Autodesk Inventor part; units mm, degrees
ref_plane "YZ Plane" through (0, 0, 0) normal (1, 0, 0) x (0, 1, 0)
ref_plane "XZ Plane" through (0, 0, 0) normal (0, 1, 0) x (-1, 0, 0)
ref_plane "XY Plane" through (0, 0, 0) normal (0, 0, 1) x (1, 0, 0)
sketch "Boceto1" plane through (0, 0, 0) normal (0, 0, 1) x (1, 0, 0)
  line L0 (0, 26.9924) -> (5, 26.9924)
  arc A0 (5, 26.9924) -> (5.5, 27.4924) centre (5, 27.4924) ccw
  line L1 (5.5, 27.4924) -> (5.5, 36.4924)
  arc A1 (6, 36.9924) -> (5.5, 36.4924) centre (6, 36.4924) ccw
  line L2 (6, 36.9924) -> (9.9731, 36.9924)
  arc A2 (10.4724, 36.4662) -> (9.9731, 36.9924) centre (9.9731, 36.4924) ccw
  line L3 (10.4724, 36.4662) -> (10.0035, 27.5185)
  arc A3 (10.0035, 27.5185) -> (10.5028, 26.9924) centre (10.5028, 27.4924) ccw
  arc A4 (23, -23.0504) -> (54.0922, -16.3077) centre (23, 52.0085) ccw
  arc A5 (106.311, -20.6517) -> (54.0922, -16.3077) centre (76.3195, -65.146) ccw
  arc A6 (106.311, -20.6517) -> (116.3303, -5.6981) centre (111.3414, -13.1888) ccw
  arc A7 (106.3579, 7.7696) -> (116.3303, -5.6981) centre (130.0298, 14.8719) ccw
  arc A8 (106.3579, 7.7696) -> (102.827, 7.7277) centre (104.6036, 6.8117) ccw
  line L4 (102.827, 7.7277) -> (98.8026, -0.0781)
  arc A9 (96.3676, -1.0494) -> (98.8026, -0.0781) centre (97.026, 0.8379) ccw
  arc A10 (96.3676, -1.0494) -> (30.1711, -1.1614) centre (63.429, -95.4689) ccw
  line L5 (13.5421, 45.9924) -> (0, 45.9924)
  arc A11 (0, 45.9924) -> (-1.9988, 43.9936) centre (0, 43.9936) ccw
  line L6 (-1.9988, 43.9936) -> (-1.9988, 28.9912)
  arc A12 (-1.9988, 28.9912) -> (0, 26.9924) centre (0, 28.9912) ccw
  circle A13 centre (111.3414, -13.1888) radius 1.9988
  circle A14 centre (31.3414, -9.1385) radius 1.9988
  line L7 (10.5028, 26.9924) -> (10.5028, -23.0504)
  line L8 (23, -23.0504) -> (13.5421, -23.0504)
  line L9 (13.5421, 45.9924) -> (27.5683, 45.9924)
  line L10 (27.5683, 45.9924) -> (27.5683, -2)
  arc A15 (27.5683, -2) -> (30.1711, -1.1614) centre (13.5421, 45.9924) ccw
  line L11 (13.5421, -23.0504) -> (10.5028, -23.0504)
  point P0 (0, 0)
extrude "Extrusión2" add sketch "Boceto1" along normal blind 5
fillet "Empalme1" radius 2 3 edges at (10.5028, -23.0504, 2.5) (27.5683, 45.9924, 2.5) (27.5683, -2, 2.5)
properties part number "soporte bobina nuevo"
Geometry check sheet. Reference: the model listing, model coordinates, mm. A direction names the side the tool comes from. Coordinates: 2 decimals unless noted, no trailing zeros. Order: outer loops, then holes, each group sorted by start corner. A loop starts at its lowest first (then second) coordinate and runs counter-clockwise, first axis right, second up. Notation, with made-up numbers: (58, 37.5) - (62, 37.5) arc R25 ccw to (62, 65.5) - close; hole circle Ø4 at (72, -37). An arc over 180 degrees is marked (long way). Answer as a JSON object with one key per item and string values. Group by question number.
Item 1: Sectioned sample at A-A, the plane y = 6.5. Record the cut outline in (x, z).
Item 2: Tool access check on faces 4 (the face through (27.568, 23, 2)), 5 (the face through (5.5, 32, 2)), 6 (the face through (10.24, 32.05, 2.46)), 7 (the face through (2, 26.992, 2)). Record the directions out of +Z, -Z, +X, -X, +Y, -Y that give a thin tool (end or side, any length) a straight path to the whole face; none if there is none.
Item 3: Sectioned sample at C-C, the plane x = 57. Record the cut outline in (y, z), and give its area (3 significant figures).
Item 4: Depth check by flat-ended pin: pin 1 Ø3.5 at (x, y) = (111.34, -13.19) entering from -Z; pin 2 Ø1.5 at (y, z) = (-4, 3) entering from -X; pin 3 Ø3 at (x, z) = (8, 3) entering from -Y; pin 4 Ø1 at (x, z) = (82, 2) entering from -Y. Enter the tip coordinate at first touch or a pass-through.
Item 5: Sectioned sample at B-B, the plane y = 15. Record the cut outline in (x, z).
Item 6: Scan lines: probe 1 along X at (y, z) = (25, 1.6); probe 2 along X at (y, z) = (43, 3.5); probe 3 along Y at (x, z) = (24.5, 1.95). Record each from-to range of solid material in increasing order.
Item 7: Sectioned sample at D-D, the plane z = 1.1. Give the number of separate pieces and of enclosed holes in the cut face, and give its area (3 significant figures).
Item 8: Draft check along X on faces 1 (the face through (62.82, 4.53, 2.46)), 2 (the face through (-1.999, 37, 2)), 3 (the face through (50, -1, 0)). Enter one of: +X half, -X half, draft (parallel to the pull), parting line (faces both ways), or undercut.
Resolved:
{
 "1": {"outline": "(10.5, 0) - (27.57, 0) - (27.57, 5) - (10.5, 5) - close; (102.19, 0) - (106.78, 0) - (106.78, 5) - (102.19, 5) - close"},
 "2": {"face 4": "+Z, -Z, +Y", "face 5": "+Z, -Z, -Y", "face 6": "+Z, -Z", "face 7": "+Z, -Z, -X, -Y"},
 "3": {"outline": "(-15.09, 0) - (4.32, 0) - (4.32, 5) - (-15.09, 5) - close", "area": "97.1 mm^2"},
 "4": {"pin 1": "through", "pin 2": "x = 10.5", "pin 3": "y = 36.99", "pin 4": "y = -11.84"},
 "5": {"outline": "(10.5, 0) - (27.57, 0) - (27.57, 5) - (10.5, 5) - close"},
 "6": {"probe 1": "10.5 to 27.57", "probe 2": "-2 to 27.57", "probe 3": "-23.04 to 45.99"},
 "7": {"separate pieces": "1", "enclosed holes": "2", "area": "3,080 mm^2"},
 "8": {"face 1": "undercut", "face 2": "-X half", "face 3": "draft"}
}
